```python
from build123d import *

# Parameters (mm, degrees)
F1_DEPTH = 9.017
F2_DEPTH = 10.795


with BuildPart() as f1:
    # F0 (on Front) → F1 (new body)
    with BuildSketch(Plane.XZ):
        with BuildLine():
            Line((-48.0792992256, 97.4998560334), (-25.5571910474, 97.1389572937))
            ThreePointArc((-25.5571910474, 97.1389572937), (-13.4866539111, 113.7481608485), (-25.5571910474, 130.3573644034))
            Line((-25.5571910474, 130.3573644034), (-25.5571910474, 113.0603018233))
            ThreePointArc((-25.5571910474, 113.0603018233), (-36.2000364442, 110.1431708658), (-46.842881841, 113.0603018233))
            Line((-46.842881841, 113.0603018233), (-46.842881841, 130.8020415732))
            ThreePointArc((-46.842881841, 130.8020415732), (-59.6904318944, 114.6049901828), (-48.0792992256, 97.4998560334))
        make_face()
    extrude(amount=F1_DEPTH)

    # F0 (on Front) → F2 (join)
    with BuildSketch(Plane.XZ):
        with BuildLine():
            Line((-27.6932814315, -29.8430773328), (-17.7972615414, -47.6693533076))
            Line((-17.7972615414, -47.6693533076), (-28.2872594454, -65.1526959162))
            Line((-28.2872594454, -65.1526959162), (-48.6732772395, -64.80976255))
            Line((-48.6732772395, -64.80976255), (-58.5692971296, -46.9834865752))
            Line((-58.5692971296, -46.9834865752), (-48.0792992256, -29.5001439666))
            Line((-48.0792992256, -29.5001439666), (-48.0792992256, -22.5995532387))
            ThreePointArc((-48.0792992256, -22.5995532387), (-53.1128208355, -69.3822114075), (-11.5496699932, -47.3264199414))
            ThreePointArc((-11.5496699932, -47.3264199414), (-15.9139266557, -32.7173447543), (-27.5764183831, -22.8960362495))
            Line((-27.5764183831, -22.8960362495), (-27.6932814315, -29.8430773328))
        make_face()
        with BuildLine():
            Line((-48.0792992256, -29.5001439666), (-27.6932814315, -29.8430773328))
            Line((-27.6932814315, -29.8430773328), (-27.5764183831, -22.8960362495))
            ThreePointArc((-27.5764183831, -22.8960362495), (-37.7981828569, -20.6955948077), (-48.0792992256, -22.5995532387))
            Line((-48.0792992256, -22.5995532387), (-48.0792992256, -29.5001439666))
        make_face()
        with BuildLine():
            ThreePointArc((-48.0792992256, -22.5995532387), (-37.7981828569, -20.6955948077), (-27.5764183831, -22.8960362495))
            Line((-27.5764183831, -22.8960362495), (-25.5571910474, 97.1389572937))
            Line((-25.5571910474, 97.1389572937), (-48.0792992256, 97.4998560334))
            Line((-48.0792992256, 97.4998560334), (-48.0792992256, -22.5995532387))
        make_face()
        with BuildLine():
            Line((-48.0792992256, 97.4998560334), (-25.5571910474, 97.1389572937))
            ThreePointArc((-25.5571910474, 97.1389572937), (-13.4866539111, 113.7481608485), (-25.5571910474, 130.3573644034))
            Line((-25.5571910474, 130.3573644034), (-25.5571910474, 113.0603018233))
            ThreePointArc((-25.5571910474, 113.0603018233), (-36.2000364442, 110.1431708658), (-46.842881841, 113.0603018233))
            Line((-46.842881841, 113.0603018233), (-46.842881841, 130.8020415732))
            ThreePointArc((-46.842881841, 130.8020415732), (-59.6904318944, 114.6049901828), (-48.0792992256, 97.4998560334))
        make_face()
    extrude(amount=F2_DEPTH)


solid = f1.part
```
Can you work these out from the model? Positions are in its coordinate system, mm. A direction names the side the tool comes from. Give positions to 0.01 mm unless a question says otherwise; leave off trailing zeros. Loops run counter-clockwise (first coordinate to the right, second up) from the corner with the lowest first, then second, coordinate; pieces in that order, holes last. Notation, with made-up numbers: M 86,84.25 L 132,84.25 A18 cw 132,89.25 Z; hole C 67,-28.75 d8. An arc over 180 degrees is marked long. Use CSV: the item, a comma, the result in double quotes. Start each with the question number.
1. If we mould it in two halves opening along Z, with no side actions, what happens to faces 4 (the face through (-13.49, -5.32, 113.44)), 5 (the face through (-36.044, -5.322, 110.144)), 6 (the face through (-25.557, -5, 122))? For each: released by +Z, released by -Z, zero draft, split by the parting line, or undercut.
2. Imagine slicing it at C-C, the plane x = -52. Write out the boundary of the cut face in (y, z) (3 decimals).
3. If I drill on L1, parallel to Z at x = -51.5, y = -8.5; L2, parallel to Z at x = -50.5, y = -3.5; L3, parallel to Z at x = -15, y = -0.75, over which ranges is the centre line in solid material (lowest first)?
4. Imagine slicing it at D-D, the plane z = 82. Write out the boundary of the cut face in (x, y) (3 decimals).
5. Imagine slicing it at B-B, the plane x = -43. Write out the boundary of the cut face in (y, z) (3 decimals).
6. For P1, Ø3, axis at y = -9, z = 35.5, coming from the +X side; P2, Ø6, axis at x = -34, y = -5, coming from the +Z side; P3, Ø1, axis at y = -5.5, z = 84, coming from the +X side, each with a flat end and sliding along its axis, tell me the tip position at first contact or that it passes through.
7. Imagine slicing it at A-A, the plane y = -6.5. Write out the boundary of the cut face in (x, z) (1 decimal), plus the area to 3 significant figures.
8. On a 3-axis mill with a long thin cutter (end or side, diameter ignored), from which of +Z, -Z, +X, -X, +Y, -Y can I reach the whole of each face in a straight line? I mean faces 1 (the face through (-48.079, -5, 38)), 2 (the face through (-46.843, -5, 122)), 3 (the face through (-22.815, -5.322, -38.631)). Say none if no direction works.
Response values:
1,face 4,"undercut"
1,face 5,"released by +Z"
1,face 6,"zero draft"
2,outline,"M -10.795,-70.096 L 0,-70.096 L 0,-58.817 L -10.795,-58.817 Z; M -10.795,-36.035 L 0,-36.035 L 0,-24.557 L -10.795,-24.557 Z; M -10.795,99.477 L 0,99.477 L 0,128.437 L -10.795,128.437 Z"
3,L1,"-70.39 to -59.72, -35.2 to -24.26, 99.15 to 128.76"
3,L2,"-70.94 to -61.52, -33.53 to -23.71, 98.57 to 129.34"
3,L3,"-60.44 to -34.22, 106.64 to 120.86"
4,outline,"M -48.079,-10.795 L -25.812,-10.795 L -25.812,0 L -48.079,0 Z"
5,outline,"M -10.795,-73.521 L 0,-73.521 L 0,-64.905 L -10.795,-64.905 Z; M -10.795,-29.586 L 0,-29.586 L 0,111.282 L -10.795,111.282 Z"
6,P1,"x = -26.57"
6,P2,"z = 110.8"
6,P3,"x = -25.77"
7,outline,"M -48.1,-22.6 A26.6 ccw long -27.6,-22.9 L -25.6,97.1 A17.5 ccw -25.6,130.4 L -25.6,113.1 A20.9 cw -46.8,113.1 L -46.8,130.8 A17.5 ccw -48.1,97.5 Z; hole M -58.6,-47 L -48.7,-64.8 L -28.3,-65.2 L -17.8,-47.7 L -27.7,-29.8 L -48.1,-29.5 Z"
7,area,"4,610 mm^2"
8,face 1,"-X, +Y, -Y"
8,face 2,"+Z, +Y, -Y"
8,face 3,"+Y, -Y"
